Verification items for the finished model (mm, model axes). A direction names the side the tool comes from. Give positions to 0.01 mm unless a question says otherwise; leave off trailing zeros. Order: outer loops, then holes, each group sorted by start corner. A loop starts at its lowest first (then second) coordinate and runs counter-clockwise, first axis right, second up. Notation, with made-up numbers: M 62,85.25 L 84,85.25 A21 cw 84,104.25 Z; hole C 10,37.25 d5. An arc over 180 degrees is marked long. Answer as a JSON object with one key per item and string values.
```python
from build123d import *

# Parameters (mm, degrees)
BOSS_EXTRUDE1_DEPTH = 19.05
SKETCH2_R           = 3.81
CUT_EXTRUDE1_DEPTH  = 89.9
SKETCH3_R           = 3.81
CUT_EXTRUDE2_DEPTH  = 89.9
SKETCH4_R           = 5.08
CUT_EXTRUDE3_DEPTH  = 20.05
FILLET1_R           = 5.08


with BuildPart() as part:
    # Sketch1 → Boss-Extrude1 (new body)
    with BuildSketch(Plane(origin=(0, 0, 0), x_dir=(0, 0, -1), z_dir=(1, 0, 0))):
        Polygon((0, 0), (0, 25.4), (-12.7, 25.4), (-12.7, 101.6), (0, 101.6), (0, 228.6), (76.2, 228.6), (76.2, 101.6), (88.9, 101.6), (88.9, 25.4), (76.2, 25.4), (76.2, 0), align=None)
    extrude(amount=BOSS_EXTRUDE1_DEPTH)

    # Sketch2 → Cut-Extrude1 (cut, through all)
    with BuildSketch(Plane.XY):
        with Locations((9.525, 114.3)):
            Circle(SKETCH2_R)
    extrude(amount=-CUT_EXTRUDE1_DEPTH, mode=Mode.SUBTRACT)

    # Sketch3 → Cut-Extrude2 (cut, through all)
    with BuildSketch(Plane.XY):
        with Locations((9.525, 12.7)):
            Circle(SKETCH3_R)
    extrude(amount=-CUT_EXTRUDE2_DEPTH, mode=Mode.SUBTRACT)

    # Sketch4 → Cut-Extrude3 (cut, through all)
    with BuildSketch(Plane(origin=(19.05, 0, 0), x_dir=(0, 0, -1), z_dir=(1, 0, 0))):
        with Locations((19.755070015, 57.415301139)):
            Circle(SKETCH4_R)
        with Locations((57.855070015, 57.415301139)):
            Circle(SKETCH4_R)
        with Locations((19.755070015, 82.815301139)):
            Circle(SKETCH4_R)
        with Locations((57.855070015, 82.815301139)):
            Circle(SKETCH4_R)
        with BuildLine():
            ThreePointArc((66.388980032, 134.027277083), (52.493130024, 162.609745262), (33.396209532, 188.013677287))
            ThreePointArc((33.396209532, 188.013677287), (26.516800005, 188.321710549), (26.208766742, 181.442301021))
            ThreePointArc((26.208766742, 181.442301021), (44.183346452, 157.531377723), (57.262526611, 130.628723299))
            ThreePointArc((57.262526611, 130.628723299), (63.525030214, 127.76477348), (66.388980032, 134.027277083))
        make_face()
    extrude(amount=-CUT_EXTRUDE3_DEPTH, mode=Mode.SUBTRACT)

    # Fillet1
    fillet1_edges = [part.edges().sort_by_distance(p)[0] for p in [
        (19.05, 25.4, -82.55),
        (0, 25.4, 6.35),
        (0, 101.6, 6.35),
        (0, 101.6, -82.55),
        (0, 25.4, -82.55),
        (19.05, 101.6, -82.55),
        (19.05, 101.6, 6.35),
        (19.05, 25.4, 6.35),
    ]]
    fillet(fillet1_edges, radius=FILLET1_R)


solid = part.part
```
Q1. Material ranges on L1, parallel to Z at x = 11.5, y = 61; L2, parallel to X at y = 114, z = -56; L3, parallel to Z at x = 17.5, y = 135, recorded low to high.
Resolved:
{"L1": "z = -88.9 to -61.45, -54.26 to -23.35, -16.16 to 12.7", "L2": "x = 0 to 5.73, 13.32 to 19.05", "L3": "z = -76.2 to -66.02, -55.56 to 0"}
Q2. Gauge pin test, flat ends, axial feed: pin 1 Ø16.5 at (y, z) = (57.42, -57.86) entering from -X; pin 2 Ø7 at (x, z) = (8.5, -83) entering from -Y; pin 3 Ø4.5 at (x, z) = (11, -80) entering from +Y; pin 4 Ø5 at (x, y) = (13, 123.5) entering from +Z. Record the tip position at first contact, or that the pin passes through.
Resolved:
{"pin 1": "stops at x = 0", "pin 2": "stops at y = 25.4", "pin 3": "stops at y = 101.6", "pin 4": "stops at z = 0"}
Q3. Tool access check on faces 1 (the face through (17.601, 100.072, 6.261)), 2 (the face through (1.449, 100.072, 6.261)), 3 (the face through (1.449, 100.072, -82.639)), 4 (the face through (9, 0, -39)), 5 (the face through (17.601, 26.928, -82.461)). Record the directions out of +Z, -Z, +X, -X, +Y, -Y that give a thin tool (end or side, any length) a straight path to the whole face; none if there is none.
Resolved:
{"face 1": "+Z, +X, +Y", "face 2": "+Z, -X, +Y", "face 3": "-Z, -X, +Y", "face 4": "+Z, -Z, +X, -X, -Y", "face 5": "-Z, +X, -Y"}
Q4. Section check D-D on z = -8. Record the cut outline in (x, y) (3 decimals), then the cut area to 3 significant figures.
Resolved:
{"outline": "M 0,0 L 19.05,0 L 19.05,228.6 L 0,228.6 Z; hole C 9.525,12.7 d7.62; hole C 9.525,114.3 d7.62", "area": "4,260 mm²"}
Q5. Section check C-C on x = 10. Record the cut outline in (y, z), then the cut area to 3 significant figures.
Resolved:
{"outline": "M 0,-76.2 L 8.92,-76.2 L 8.92,0 L 0,0 Z; M 16.48,-76.2 L 25.4,-76.2 L 25.4,-88.9 L 101.6,-88.9 L 101.6,-76.2 L 110.52,-76.2 L 110.52,0 L 101.6,0 L 101.6,12.7 L 25.4,12.7 L 25.4,0 L 16.48,0 Z; M 118.08,-76.2 L 228.6,-76.2 L 228.6,0 L 118.08,0 Z; hole C 57.42,-57.86 d10.16; hole C 57.42,-19.76 d10.16; hole C 82.82,-57.86 d10.16; hole C 82.82,-19.76 d10.16; hole M 130.63,-57.26 A4.87 ccw 134.03,-66.39 A165.71 ccw 188.01,-33.4 A4.87 ccw 181.44,-26.21 A155.97 cw Z", "area": "17,200 mm²"}
Q6. Release check for a two-part mould opening along Y. For faces 6 (the face through (9.66, 62.45, -57.19)), 7 (the face through (9, 101.6, -82)), 8 (the face through (9, 25.4, -83)), 9 (the face through (9.658, 188.393, -26.597)) record: +Y half, -Y half, draft (parallel to the pull), parting line (faces both ways), or undercut.
Resolved:
{"face 6": "undercut", "face 7": "+Y half", "face 8": "-Y half", "face 9": "undercut"}
Q7. Section check B-B on y = 12.7. Record the cut outline in (x, z) (3 decimals).
Resolved:
{"outline": "M 0,-76.2 L 5.715,-76.2 L 5.715,0 L 0,0 Z; M 13.335,-76.2 L 19.05,-76.2 L 19.05,0 L 13.335,0 Z"}
Q8. Section check A-A on z = -19. Record the cut outline in (x, y) (3 decimals), then the cut area to 3 significant figures.
Resolved:
{"outline": "M 0,0 L 19.05,0 L 19.05,52.392 L 0,52.392 Z; M 0,62.439 L 19.05,62.439 L 19.05,77.792 L 0,77.792 Z; M 0,87.839 L 19.05,87.839 L 19.05,228.6 L 0,228.6 Z; hole C 9.525,12.7 d7.62; hole C 9.525,114.3 d7.62", "area": "3,880 mm²"}
